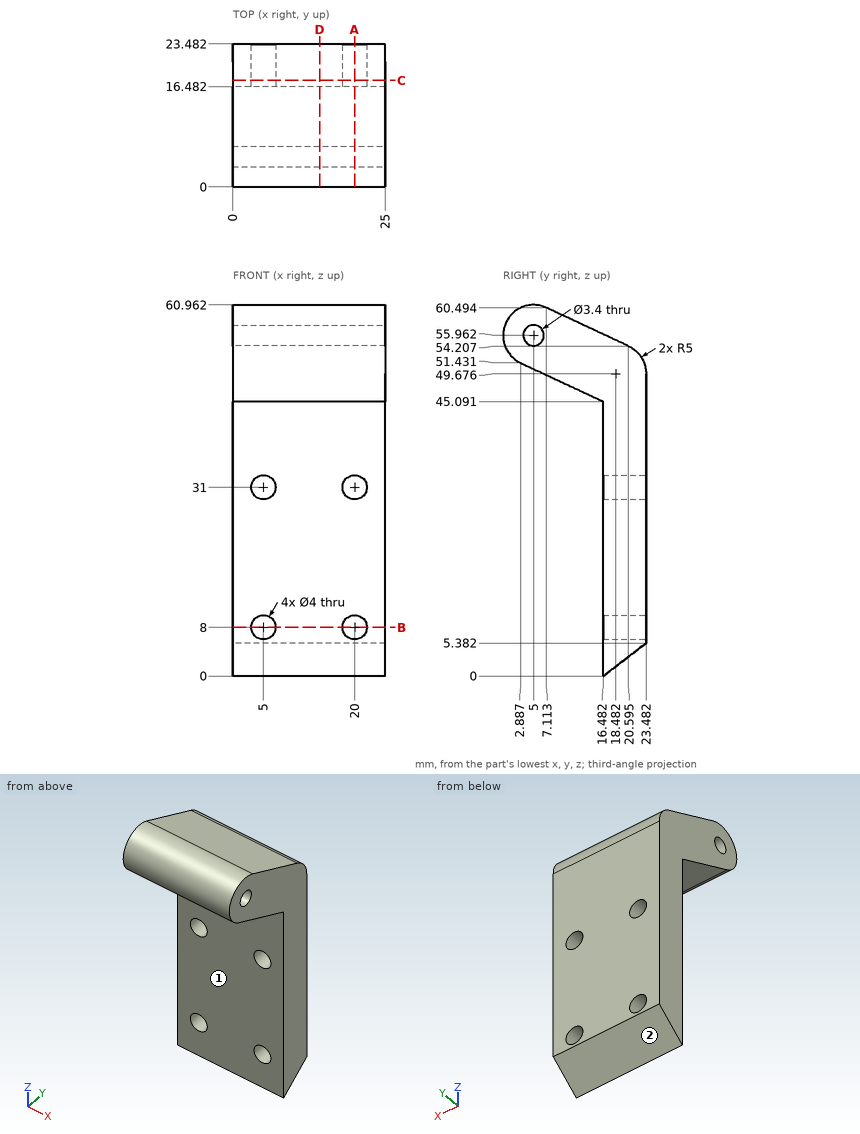
Here's the drawing with two shaded views (mm, measured from the low corner). I have some questions. A direction names the side the tool comes from. Give positions to 0.01 mm unless a question says otherwise; leave off trailing zeros. Write each loop counter-clockwise with the first axis right and the second up, starting at its lowest first coordinate (ties: lowest second). Pieces come first, ordered by that corner, then holes. Notation, with made-up numbers: (76, -37) - (92, -37) arc R14 cw to (92, -31) - close; hole circle Ø6 at (69.5, -13). An arc over 180 degrees is marked (long way). Write item = value, one per line. Start each with the question number.
1. For pin 1 (3 mm diameter, centred on x = 5, y = 7.5, fed in from +Z); pin 2 (6 mm diameter, centred on x = 19.5, y = 8, fed in from -Z); pin 3 (6 mm diameter, centred on x = 15, z = 54.5, fed in from +Y), each with a flat end and sliding along its axis, tell me the tip position at first contact or that it passes through.
2. Please list where these lines run through material, in increasing order: line 1 (X direction, y = 21.5, z = 8); line 2 (Z direction, x = 5, y = 21.75); line 3 (Z direction, x = 4, y = 18.25).
3. On a 3-axis mill with a long thin cutter (end or side, diameter ignored), from which of +Z, -Z, +X, -X, +Y, -Y can I reach the whole of each face in a straight line? I mean the marked faces 1 and 2. Say none if no direction works.
4. Imagine slicing it at A-A (x = 20). Please give me the cut outline in (y, z) (1 decimal), and give its area (3 significant figures).
5. Imagine slicing it at B-B (z = 8). Please give me the cut outline in (x, y).
6. Imagine slicing it at C-C (y = 17.5). Please give me the cut outline in (x, z), and give its area (3 significant figures).
7. Imagine slicing it at D-D (x = 14.25). Please give me the cut outline in (y, z) (1 decimal).
Worked answers:
q1.pin_1 = 60.86
q1.pin_2 = 47.65
q1.pin_3 = 23.14
q2.line_1 = 0 to 3, 7 to 18, 22 to 25
q2.line_2 = 4.05 to 6, 10 to 29, 33 to 53.46
q2.line_3 = 1.36 to 6.27, 9.73 to 29.27, 32.73 to 55.3
q3.face_1 = -Z, +X, -X, -Y
q3.face_2 = -Z, +X, -X, +Y
q4.outline = (2.9, 51.4) - (16.5, 45.1) - (16.5, 33) - (23.5, 33) - (23.5, 49.7) arc R5 ccw to (20.6, 54.2) - (7.1, 60.5) arc R5 ccw to start; (16.5, 0) - (23.5, 5.4) - (23.5, 6) - (16.5, 6) - close; (16.5, 10) - (23.5, 10) - (23.5, 29) - (16.5, 29) - close; hole circle Ø3.4 at (5, 56)
q4.area = 462 mm2
q5.outline = (0, 16.48) - (3, 16.48) - (3, 23.48) - (0, 23.48) - close; (7, 16.48) - (18, 16.48) - (18, 23.48) - (7, 23.48) - close; (22, 16.48) - (25, 16.48) - (25, 23.48) - (22, 23.48) - close
q6.outline = (0, 0.78) - (25, 0.78) - (25, 55.65) - (0, 55.65) - close; hole circle Ø4 at (5, 8); hole circle Ø4 at (5, 31); hole circle Ø4 at (20, 8); hole circle Ø4 at (20, 31)
q6.area = 1,320 mm2
q7.outline = (2.9, 51.4) - (16.5, 45.1) - (16.5, 0) - (23.5, 5.4) - (23.5, 49.7) arc R5 ccw to (20.6, 54.2) - (7.1, 60.5) arc R5 ccw to start; hole circle Ø3.4 at (5, 56)
